from build123d import *

# Parameters (mm, degrees)
CYLINDER005_R     = 6.5
CYLINDER005_DEPTH = 10
CYLINDER004_R     = 8.2
CYLINDER004_DEPTH = 5
BOX_W             = 10
BOX_H             = 26.4
BOX_DEPTH         = 26.4
FILLET_R          = 10


with BuildPart() as bring_holder_hole:
    # Cylinder005 → Cylinder005 (new body)
    with BuildSketch(Plane(origin=(0, 0, 0), x_dir=(0, 0, -1), z_dir=(1, 0, 0))):
        Circle(CYLINDER005_R)
    extrude(amount=CYLINDER005_DEPTH)


with BuildPart() as bring_holder_extract:
    # Cylinder004 → Cylinder004 (new body)
    with BuildSketch(Plane(origin=(0, 0, 0), x_dir=(0, 0, -1), z_dir=(1, 0, 0))):
        Circle(CYLINDER004_R)
    extrude(amount=CYLINDER004_DEPTH)

    # Fusion001: union bring holder hole
    add(bring_holder_hole.part)


with BuildPart() as bring_holder_cut_clone:
    # Box → Box (new body)
    with BuildSketch(Plane(origin=(0, -13.2, -13.2), x_dir=(1, 0, 0), z_dir=(0, 0, 1))):
        with Locations((5, 13.2)):
            Rectangle(BOX_W, BOX_H)
    extrude(amount=BOX_DEPTH)

    # Fillet
    fillet_edges = [bring_holder_cut_clone.edges().sort_by_distance(p)[0] for p in [
        (5, -13.2, 13.2),
        (5, 13.2, -13.2),
        (5, 13.2, 13.2),
    ]]
    fillet(fillet_edges, radius=FILLET_R)

    # Cut023015003: cut bring holder extract
    add(bring_holder_extract.part, mode=Mode.SUBTRACT)


with BuildPart() as bring_holder_cut_clone_1:
    # Cut023015003 placement: moved
    add(bring_holder_cut_clone.part.moved(Location((-5, 26, 13.2))))


with BuildPart() as bring_holder_cut_clone_2:
    # Clone002 placement: moved
    add(bring_holder_cut_clone_1.part.moved(Location((0, 0, -6.2))))


with BuildPart() as bring_holder_cut_clone_3:
    # Body003 placement: moved
    add(bring_holder_cut_clone_2.part.moved(Location((0, 8, 9))))


solid = bring_holder_cut_clone_3.part
Input: part model. Units: mm. Frame: model coordinates. A direction names the side the tool comes from. Coordinates: 2 decimals unless noted, no trailing zeros. Loops run counter-clockwise (first coordinate to the right, second up) from the corner with the lowest first, then second, coordinate; pieces in that order, holes last.
Q1. Cut plane C-C (x = 1.75). Output: boundary loops of the cut face in (y, z).
Q2. Cut plane B-B (z = 16). Output: boundary loops of the cut face in (x, y).
Q3. Set-up query: faces 4 (the face through (0, 34, 29.2)), 5 (the face through (0, 38, 22)). Return all of +Z, -Z, +X, -X, +Y, -Y with unobstructed straight access to the full face (end or side cutting, diameter ignored); none if empty.
Q4. Cut plane A-A (y = 34). Output: boundary loops of the cut face in (x, z).
Q5. Draft query along Z for faces 1 (the face through (2.465, 38.393, 20.791)), 2 (the face through (0, 29, 2.8)), 3 (the face through (0.07, 23.65, 26.19)). Return one class per face: +Z half, -Z half, draft (parallel to the pull), parting line (faces both ways), or undercut.
Q6. Material intervals for line 1 (Z direction, x = 1.75, y = 34); line 2 (Y direction, x = -1.45, z = 16); line 3 (Y direction, x = 2.35, z = 16), sorted ascending.
Q7. Cut plane D-D (y = 45). Output: boundary loops of the cut face in (x, z), then the cut area to 3 significant figures.
Q8. Contact query for flat-ended pins moving along their axis: pin 1 (1 mm diameter, centred on y = 28.5, z = 13.5, fed in from -X); pin 2 (1.5 mm diameter, centred on x = 4, y = 29, fed in from +Z). Output: stop coordinate, or through.
Working result:
1. outline: (20.8, 2.8) - (37.2, 2.8) arc R10 ccw to (47.2, 12.8) - (47.2, 19.2) arc R10 ccw to (37.2, 29.2) - (30.8, 29.2) arc R10 ccw to (20.8, 19.2) - close; hole circle Ø13 at (34, 16)
2. outline: (-5, 20.8) - (5, 20.8) - (5, 27.5) - (0, 27.5) - (0, 25.8) - (-5, 25.8) - close; (-5, 42.2) - (0, 42.2) - (0, 40.5) - (5, 40.5) - (5, 47.2) - (-5, 47.2) - close
3. face 4: +Z, +X, -X, +Y, -Y
3. face 5: -X
4. outline: (-5, 2.8) - (5, 2.8) - (5, 9.5) - (0, 9.5) - (0, 7.8) - (-5, 7.8) - close; (-5, 24.2) - (0, 24.2) - (0, 22.5) - (5, 22.5) - (5, 29.2) - (-5, 29.2) - close
5. face 1: undercut
5. face 2: -Z half
5. face 3: +Z half
6. line 1: z = 2.8 to 9.5, 22.5 to 29.2
6. line 2: y = 20.8 to 25.8, 42.2 to 47.2
6. line 3: y = 20.8 to 27.5, 40.5 to 47.2
7. outline: (-5, 6.54) - (5, 6.54) - (5, 25.46) - (-5, 25.46) - close
7. area: 189 mm2
8. pin 1: stops at x = 0
8. pin 2: stops at z = 29.14
